from build123d import *

# Parameters (mm, degrees)
BOSS_EXTRUDE1_DEPTH = 400
FILLET1_R           = 1
FILLET2_R           = 1


with BuildPart() as part:
    # Sketch1 → Boss-Extrude1 (new body)
    with BuildSketch(Plane.XY):
        Polygon((-11, 5), (-11, 0), (11, 0), (11, 5), (20.5, 5), (20.5, -5), (-20.5, -5), (-20.5, 5), align=None)
    extrude(amount=BOSS_EXTRUDE1_DEPTH)

    # Fillet1
    fillet1_edges = [part.edges().sort_by_distance(p)[0] for p in [
        (20.5, 5, 200),
        (20.5, -5, 200),
        (-20.5, -5, 200),
        (-20.5, 5, 200),
        (-11, 5, 200),
        (11, 5, 200),
    ]]
    fillet(fillet1_edges, radius=FILLET1_R)

    # Fillet2
    fillet2_edges = [part.edges().sort_by_distance(p)[0] for p in [
        (0, 0, 400),
        (-11, 2, 400),
        (11, 2, 0),
        (11, 2, 400),
        (15.75, 5, 0),
        (20.5, 0, 0),
        (0, -5, 0),
        (-20.5, 0, 0),
        (-15.75, 5, 0),
        (20.207106781, 4.707106781, 0),
        (-20.207106781, 4.707106781, 0),
        (-20.207106781, -4.707106781, 0),
        (20.207106781, -4.707106781, 0),
        (-11.292893219, 4.707106781, 0),
        (11.292893219, 4.707106781, 0),
        (15.75, 5, 400),
        (-15.75, 5, 400),
        (-20.5, 0, 400),
        (0, -5, 400),
        (20.5, 0, 400),
        (20.207106781, 4.707106781, 400),
        (-20.207106781, 4.707106781, 400),
        (-20.207106781, -4.707106781, 400),
        (20.207106781, -4.707106781, 400),
        (-11.292893219, 4.707106781, 400),
        (11.292893219, 4.707106781, 400),
        (-11, 2, 0),
        (0, 0, 0),
    ]]
    fillet(fillet2_edges, radius=FILLET2_R)


solid = part.part
Build history of the part. All positions in model axes, mm. Coordinates: 2 decimals unless noted, no trailing zeros. Write each loop counter-clockwise with the first axis right and the second up, starting at its lowest first coordinate (ties: lowest second). Pieces come first, ordered by that corner, then holes.
(1) Pin check, flat tips, straight feed: pin 1 Ø2 at (x, y) = (-3.5, 0.5) entering from -Z; pin 2 Ø5 at (x, z) = (-4, 84.5) entering from +Y; pin 3 Ø1.5 at (x, y) = (9.5, 0.5) entering from +Z. Stop position of each tip, or through.
(2) Cut at B-B on z = 123. List the corners of the cut face in (x, y), and give its area (3 significant figures).
(3) Mould opens along X. For faces 1 (the flat face through (20.5, 0, 197)), 2 (the flat face through (0, 0, 197)), 3 (the flat face through (0, -5, 197)), 4 (the flat face through (-20.5, 0, 197)) say: pulls with the +X half, pulls with the -X half, needs draft (parallel to the pull), parting line crosses it, or undercut.
(4) Cut at A-A on y = 2. List the corners of the cut face in (x, z).
(5) Cut at C-C on x = 4.5. List the corners of the cut face in (y, z).
(6) Drill centre lines: line 1 (X direction, y = 3.25, z = 352.5); line 2 (X direction, y = -4.25, z = 384.5); line 3 (Y direction, x = 7.5, z = 112). Where is each one in solid material? Low to high.
Working result:
1. pin 1: stops at z = 0.13
1. pin 2: stops at y = 0
1. pin 3: stops at z = 399.66
2. outline: (-20.5, -4) arc R1 ccw to (-19.5, -5) - (19.5, -5) arc R1 ccw to (20.5, -4) - (20.5, 4) arc R1 ccw to (19.5, 5) - (12, 5) arc R1 ccw to (11, 4) - (11, 0) - (-11, 0) - (-11, 4) arc R1 ccw to (-12, 5) - (-19.5, 5) arc R1 ccw to (-20.5, 4) - close
2. area: 299 mm2
3. face 1: pulls with the +X half
3. face 2: undercut
3. face 3: needs draft
3. face 4: pulls with the -X half
4. outline: (-20.5, 1) arc R1 ccw to (-19.5, 0) - (-12, 0) arc R1 ccw to (-11, 1) - (-11, 399) arc R1 ccw to (-12, 400) - (-19.5, 400) arc R1 ccw to (-20.5, 399) - close; (11, 1) arc R1 ccw to (12, 0) - (19.5, 0) arc R1 ccw to (20.5, 1) - (20.5, 399) arc R1 ccw to (19.5, 400) - (12, 400) arc R1 ccw to (11, 399) - close
5. outline: (-5, 1) arc R1 ccw to (-4, 0) - (-1, 0) arc R1 ccw to (0, 1) - (0, 399) arc R1 ccw to (-1, 400) - (-4, 400) arc R1 ccw to (-5, 399) - close
6. line 1: x = -20.5 to -11, 11 to 20.5
6. line 2: x = -20.47 to 20.47
6. line 3: y = -5 to 0
